Autodesk Inventor part; units mm, degrees
ref_plane "YZ Plane" through (0, 0, 0) normal (1, 0, 0) x (0, 1, 0)
ref_plane "XZ Plane" through (0, 0, 0) normal (0, 1, 0) x (-1, 0, 0)
ref_plane "XY Plane" through (0, 0, 0) normal (0, 0, 1) x (1, 0, 0)
sketch "Esquisse1" plane through (0, 0, 0) normal (0, 1, 0) x (-1, 0, 0)
  line L0 (7.7669, 18.1799) -> (-22.2331, 18.1799)
  line L1 (-22.2331, 18.1799) -> (-22.2331, -11.8201)
  line L2 (-22.2331, -11.8201) -> (7.7669, -11.8201)
  line L3 (7.7669, -11.8201) -> (7.7669, 18.1799)
  point P0 (0, 0)
  dimension "d0" = 30
  dimension "d1" = 30
extrude "Extrusion1" add sketch "Esquisse1" along normal blind 9
sketch "Esquisse2" plane through (0, 9, 0) normal (0, 1, 0) x (1, 0, 0)
  circle A0 centre (-3.7669, -14.1799) radius 1.5
  circle A1 centre (18.2331, 7.8201) radius 1.5
  line L0 (-7.7669, 11.8201) -> (-7.7669, -18.1799)
  line L1 (-7.7669, -18.1799) -> (22.2331, -18.1799)
  line L2 (22.2331, 11.8201) -> (-7.7669, 11.8201)
  line L3 (22.2331, -18.1799) -> (22.2331, 11.8201)
  point P0 (0, 0)
  dimension "d4" = 3
  dimension "d5" = 3
  dimension "d6" = 4
  dimension "d8" = 4
  dimension "d9" = 4
  dimension "d13" = 4
extrude "Extrusion2" cut sketch "Esquisse2" against normal blind 10 contours A0 | A1
fillet "Congé1" radius 1 12 edges at (7.2331, 9, 18.1799) (22.2331, 9, 3.1799) (7.2331, 9, -11.8201) (-7.7669, 9, 3.1799) (-7.7669, 0, 3.1799) (7.2331, 0, -11.8201) (22.2331, 0, 3.1799) (7.2331, 0, 18.1799) (22.2331, 4.5, 18.1799) (22.2331, 4.5, -11.8201) (-7.7669, 4.5, -11.8201) (-7.7669, 4.5, 18.1799)
properties part number "calle-patin"
Model file for the job. Use its own axes, mm. Give positions to 0.01 mm unless a question says otherwise; leave off trailing zeros. Order: outer loops, then holes, each group sorted by start corner. A loop starts at its lowest first (then second) coordinate and runs counter-clockwise, first axis right, second up. Notation, with made-up numbers: M -13,42 L 26,42 A30 cw 26,75 Z; hole C 15.5,-7 d3. An arc over 180 degrees is marked long. Put each result on its own line as item: value. Start each with the question number.
(1) Pin check, flat tip, straight feed: pin 1 Ø3.5 at (x, z) = (18.23, -7.82) entering from +Y. Stop position of the tip, or through.
(2) Band-saw the part on C-C on x = -2.75. Give the cut face in (y, z), then the cut area to 3 significant figures.
(3) Band-saw the part on B-B on y = 7.5. Give the cut face in (x, z).
(4) Band-saw the part on A-A on x = 18. Give the cut face in (y, z).
(5) Pull direction X, two halves, no side cores. Call faces 1 (the face through (16.735, 4.563, -7.886)), 2 (the face through (-7.47, 8.71, 3.38)), 3 (the face through (21.95, 4.55, -11.52)), 4 (the face through (7.429, 8.715, 17.879)): released by +X, released by -X, zero draft, split by the parting line, or undercut.
(6) Drill centre lines: L1, parallel to Z at x = -3.75, y = 1.25; L2, parallel to X at y = 7.5, z = 13.5; L3, parallel to Z at x = 17.75, y = 8. Where is each one in solid material? Low to high. Write a range as [from, to].
Results below:
1. pin 1: stops at y = 9
2. outline: M 0,-10.82 A1 ccw 1,-11.82 L 8,-11.82 A1 ccw 9,-10.82 L 9,13.08 L 0,13.08 Z; M 0,15.28 L 9,15.28 L 9,17.18 A1 ccw 8,18.18 L 1,18.18 A1 ccw 0,17.18 Z
2. area: 249 mm2
3. outline: M -7.77,-10.82 A1 ccw -6.77,-11.82 L 21.23,-11.82 A1 ccw 22.23,-10.82 L 22.23,17.18 A1 ccw 21.23,18.18 L -6.77,18.18 A1 ccw -7.77,17.18 Z; hole C -3.77,14.18 d3; hole C 18.23,-7.82 d3
4. outline: M 0,-10.82 A1 ccw 1,-11.82 L 8,-11.82 A1 ccw 9,-10.82 L 9,-9.3 L 0,-9.3 Z; M 0,-6.34 L 9,-6.34 L 9,17.18 A1 ccw 8,18.18 L 1,18.18 A1 ccw 0,17.18 Z
5. face 1: undercut
5. face 2: released by -X
5. face 3: released by +X
5. face 4: zero draft
6. L1: z = [-11.82, 12.68], [15.68, 18.18]
6. L2: x = [-7.77, -5.1], [-2.43, 22.23]
6. L3: z = [-11.82, -9.24], [-6.4, 18.18]
